```python
from build123d import *

# Parameters (mm, degrees)
SKETCH1_W               = 12
SKETCH1_H               = 12
SKETCH1_R               = 5.5
BOSS_EXTRUDE1_DEPTH     = 2
BOSS_EXTRUDE1_2_DEPTH   = 2
BOSS_EXTRUDE1_3_DEPTH   = 2
BOSS_EXTRUDE1_4_DEPTH   = 2
BOSS_EXTRUDE1_5_DEPTH   = 2
BOSS_EXTRUDE1_6_DEPTH   = 2
BOSS_EXTRUDE2_START     = -10
BOSS_EXTRUDE2_OUTLINE_R = 1.7
BOSS_EXTRUDE2_DEPTH     = 10
CUT_EXTRUDE1_DEPTH      = 1


# Read off the part's stored shape, not the designer's step: Boss-Extrude2
with BuildPart() as part:
    # Sketch1 → Boss-Extrude1 (new body)
    with BuildSketch(Plane(origin=(0, 0, 0), x_dir=(1, 0, 0), z_dir=(0, 1, 0))):
        with Locations((13.686388819, -10.664882883)):
            Rectangle(SKETCH1_W, SKETCH1_H)
        with Locations(Location((13.686388819, -10.664882883, 0), (0, 0, 270))):
            Circle(SKETCH1_R, mode=Mode.SUBTRACT)
    extrude(amount=-BOSS_EXTRUDE1_DEPTH)



with BuildPart() as body_2:
    # Sketch1 → Boss-Extrude1 2 (new body)
    with BuildSketch(Plane(origin=(0, 0, 0), x_dir=(1, 0, 0), z_dir=(0, 1, 0))):
        with Locations((-1.113611181, -10.664882883)):
            Rectangle(SKETCH1_W, SKETCH1_H)
        with Locations(Location((-1.113611181, -10.664882883, 0), (0, 0, 270))):
            Circle(SKETCH1_R, mode=Mode.SUBTRACT)
    extrude(amount=-BOSS_EXTRUDE1_2_DEPTH)


with BuildPart() as body_3:
    # Sketch1 → Boss-Extrude1 3 (new body)
    with BuildSketch(Plane(origin=(0, 0, 0), x_dir=(1, 0, 0), z_dir=(0, 1, 0))):
        with Locations((6.28638882, -23.664882883)):
            Rectangle(SKETCH1_W, SKETCH1_H)
        with Locations(Location((6.28638882, -23.664882883, 0), (0, 0, 270))):
            Circle(SKETCH1_R, mode=Mode.SUBTRACT)
    extrude(amount=-BOSS_EXTRUDE1_3_DEPTH)


with BuildPart() as body_4:
    # Sketch1 → Boss-Extrude1 4 (new body)
    with BuildSketch(Plane(origin=(0, 0, 0), x_dir=(1, 0, 0), z_dir=(0, 1, 0))):
        with Locations((21.08638882, -23.664882883)):
            Rectangle(SKETCH1_W, SKETCH1_H)
        with Locations(Location((21.08638882, -23.664882883, 0), (0, 0, 270))):
            Circle(SKETCH1_R, mode=Mode.SUBTRACT)
    extrude(amount=-BOSS_EXTRUDE1_4_DEPTH)


with BuildPart() as body_5:
    # Sketch1 → Boss-Extrude1 5 (new body)
    with BuildSketch(Plane(origin=(0, 0, 0), x_dir=(1, 0, 0), z_dir=(0, 1, 0))):
        with Locations((35.88638882, -23.664882883)):
            Rectangle(SKETCH1_W, SKETCH1_H)
        with Locations(Location((35.88638882, -23.664882883, 0), (0, 0, 270))):
            Circle(SKETCH1_R, mode=Mode.SUBTRACT)
    extrude(amount=-BOSS_EXTRUDE1_5_DEPTH)


with BuildPart() as body_6:
    # Sketch1 → Boss-Extrude1 6 (new body)
    with BuildSketch(Plane(origin=(0, 0, 0), x_dir=(1, 0, 0), z_dir=(0, 1, 0))):
        with Locations((28.486388819, -10.664882883)):
            Rectangle(SKETCH1_W, SKETCH1_H)
        with Locations(Location((28.486388819, -10.664882883, 0), (0, 0, 270))):
            Circle(SKETCH1_R, mode=Mode.SUBTRACT)
    extrude(amount=-BOSS_EXTRUDE1_6_DEPTH)


with BuildPart() as part_1:
    add(part.part)

    add(body_2.part)  # Boss-Extrude2 merges body 2

    add(body_3.part)  # Boss-Extrude2 merges body 3

    add(body_4.part)  # Boss-Extrude2 merges body 4

    add(body_5.part)  # Boss-Extrude2 merges body 5

    add(body_6.part)  # Boss-Extrude2 merges body 6
    # Boss-Extrude2 outline → Boss-Extrude2 (add)
    with BuildSketch(Plane(origin=(0, 0, 0), x_dir=(1, 0, 0), z_dir=(0, 1, 0)).offset(BOSS_EXTRUDE2_START)):
        Polygon((22.486388819, -4.664882883), (25.986388819, -4.664882883), (25.986388819, -4.164882883), (16.186388819, -4.164882883), (16.186388819, -4.664882883), (19.686388819, -4.664882883), (19.686388819, -16.664882883), (7.686388819, -16.664882883), (7.686388819, -4.664882883), (11.186388819, -4.664882883), (11.186388819, -4.164882883), (1.386388819, -4.164882883), (1.386388819, -4.664882883), (4.886388819, -4.664882883), (4.886388819, -16.664882883), (-7.113611181, -16.664882883), (-7.113611181, -4.664882883), (-3.613611181, -4.664882883), (-3.613611181, -4.164882883), (-18.613611181, -4.164883527), (-18.613611181, -30.164882449), (3.78638882, -30.164882883), (3.78638882, -29.664882883), (0.28638882, -29.664882883), (0.28638882, -17.664882883), (12.28638882, -17.664882883), (12.28638882, -29.664882883), (8.78638882, -29.664882883), (8.78638882, -30.164882883), (18.58638882, -30.164882883), (18.58638882, -29.664882883), (15.08638882, -29.664882883), (15.08638882, -17.664882883), (27.08638882, -17.664882883), (27.08638882, -29.664882883), (23.58638882, -29.664882883), (23.58638882, -30.164882883), (33.38638882, -30.164882883), (33.38638882, -29.664882883), (29.88638882, -29.664882883), (29.88638882, -17.664882883), (41.88638882, -17.664882883), (41.88638882, -29.664882883), (38.38638882, -29.664882883), (38.38638882, -30.164882883), (53.38638882, -30.164882883), (53.38638882, -4.164882883), (30.986388819, -4.164882883), (30.986388819, -4.664882883), (34.486388819, -4.664882883), (34.486388819, -16.664882883), (22.486388819, -16.664882883), align=None)
        with Locations((-13.613611181, -17.164882988)):
            Circle(BOSS_EXTRUDE2_OUTLINE_R, mode=Mode.SUBTRACT)
        with Locations((48.386388819, -17.164882988)):
            Circle(BOSS_EXTRUDE2_OUTLINE_R, mode=Mode.SUBTRACT)
    extrude(amount=BOSS_EXTRUDE2_DEPTH)

    # Sketch2 → Cut-Extrude1 (cut)
    with BuildSketch(Plane.XZ.offset(10)):
        Polygon((-11.090813446, 25.393846705), (-9.544018575, 25.393846705), (-9.544018575, 25.068205679), (-10.805877549, 25.068205679), (-10.805877549, 24.091282602), (-9.544018575, 24.091282602), (-9.544018575, 23.765641577), (-10.805877549, 23.765641577), (-10.805877549, 22.218846705), (-11.090813446, 22.218846705), align=None)
        with BuildLine():
            Line((-8.852031395, 24.416923628), (-9.136967293, 24.416923628))
            add(Edge.make_bspline(
                [(-9.136967293, 24.416923628), (-9.135110232, 24.454725076), (-9.131463015, 24.528966114), (-9.114383067, 24.637209944), (-9.089943843, 24.74067394), (-9.055389453, 24.838527362), (-9.012475901, 24.931635423), (-8.961013662, 25.019628294), (-8.90005924, 25.102170301), (-8.830928846, 25.178496252), (-8.755845866, 25.248516405), (-8.674832621, 25.308982233), (-8.589701775, 25.360070406), (-8.500711605, 25.402779818), (-8.406858094, 25.434838107), (-8.30899293, 25.45862488), (-8.206686142, 25.472936279), (-8.136981265, 25.474474599), (-8.101530594, 25.475256961)],
                knots=[0, 0, 0, 0, 1.10065271, 2.161652631, 3.183658789, 4.190468796, 5.17591951, 6.163126047, 7.15150782, 8.156236427, 9.156009102, 10.134482811, 11.092018607, 12.041330605, 13.001268258, 13.972401359, 14.968799086, 16, 16, 16, 16], degree=3))
            add(Edge.make_bspline(
                [(-8.101530594, 25.475256961), (-8.066716198, 25.474441933), (-7.998307154, 25.472840431), (-7.898465184, 25.459087212), (-7.803417209, 25.437546568), (-7.713349021, 25.407324726), (-7.628979234, 25.366698853), (-7.549674044, 25.3178968), (-7.474489308, 25.261454524), (-7.406810297, 25.195002851), (-7.344663683, 25.124062116), (-7.291049494, 25.048326661), (-7.245136124, 24.97010438), (-7.206865872, 24.888798797), (-7.178693517, 24.803644364), (-7.157304714, 24.71588083), (-7.145214846, 24.624599752), (-7.143359355, 24.562817376), (-7.142416011, 24.531406801)],
                knots=[0, 0, 0, 0, 1.111607364, 2.184268762, 3.212621178, 4.221274766, 5.211760367, 6.196651075, 7.1921475, 8.207485113, 9.220403448, 10.201281604, 11.166441695, 12.114753415, 13.065576456, 14.026450734, 14.996634279, 16, 16, 16, 16], degree=3))
            add(Edge.make_bspline(
                [(-7.142416011, 24.531406801), (-7.143946038, 24.48718376), (-7.146979244, 24.399513729), (-7.173155489, 24.270514062), (-7.21359782, 24.145414473), (-7.262649782, 24.044740618), (-7.31219844, 23.964025865), (-7.355904397, 23.896973819), (-7.408203317, 23.825466998), (-7.468616685, 23.748785207), (-7.536233124, 23.666693885), (-7.611539287, 23.579159348), (-7.695110449, 23.487111285), (-7.753764656, 23.424241012), (-7.784157797, 23.391663211)],
                knots=[0, 0, 0, 0, 1.184203166, 2.347625244, 3.513805382, 4.700623107, 5.337941753, 6.051866363, 6.845199593, 7.711357327, 8.668078039, 9.695487809, 10.805859518, 12, 12, 12, 12], degree=3))
            Line((-7.784157797, 23.391663211), (-8.578543815, 22.544487731))
            Line((-8.578543815, 22.544487731), (-7.101710882, 22.544487731))
            Line((-7.101710882, 22.544487731), (-7.101710882, 22.218846705))
            Line((-7.101710882, 22.218846705), (-9.259082677, 22.218846705))
            Line((-9.259082677, 22.218846705), (-8.027752549, 23.532859125))
            add(Edge.make_bspline(
                [(-8.027752549, 23.532859125), (-7.997773395, 23.564154017), (-7.940189574, 23.624265101), (-7.858743951, 23.712024786), (-7.785592869, 23.793440441), (-7.720262805, 23.868358238), (-7.664170983, 23.937874018), (-7.614394029, 23.999736356), (-7.574510957, 24.056663607), (-7.531226277, 24.122649736), (-7.489303594, 24.203215195), (-7.453278814, 24.301670756), (-7.431312487, 24.403023335), (-7.428677386, 24.471514469), (-7.427351908, 24.505966096)],
                knots=[0, 0, 0, 0, 1.329631726, 2.553950428, 3.673215718, 4.687767853, 5.603093632, 6.413772471, 7.123043292, 7.734684054, 8.834405432, 9.900288307, 10.943827018, 12, 12, 12, 12], degree=3))
            add(Edge.make_bspline(
                [(-7.427351908, 24.505966096), (-7.427928617, 24.527629936), (-7.4290652, 24.570325205), (-7.439096111, 24.632923286), (-7.454254927, 24.693307081), (-7.475976697, 24.751662329), (-7.504648526, 24.807402313), (-7.539549378, 24.860594884), (-7.579817506, 24.912019874), (-7.626400444, 24.960237509), (-7.677573751, 25.004398317), (-7.731634249, 25.043518023), (-7.7888297, 25.076210645), (-7.848918954, 25.103010817), (-7.911734487, 25.124034199), (-7.977397792, 25.138601624), (-8.045727435, 25.147747878), (-8.092384963, 25.148985376), (-8.116158999, 25.149615936)],
                knots=[0, 0, 0, 0, 0.991446411, 1.95395049, 2.89581595, 3.838931463, 4.798493298, 5.75982156, 6.748411868, 7.785213223, 8.824556874, 9.840280684, 10.836137867, 11.835679398, 12.848801643, 13.863922112, 14.911575587, 16, 16, 16, 16], degree=3))
            add(Edge.make_bspline(
                [(-8.116158999, 25.149615936), (-8.140988255, 25.148967299), (-8.189748813, 25.147693485), (-8.26133965, 25.138782925), (-8.329634605, 25.123410627), (-8.394805474, 25.102386072), (-8.456962527, 25.07566296), (-8.515803481, 25.042378306), (-8.571196245, 25.002660423), (-8.623244948, 24.957629347), (-8.671200129, 24.907493737), (-8.713334081, 24.851604699), (-8.75014958, 24.790982687), (-8.782270813, 24.725791273), (-8.808356332, 24.655438916), (-8.828289118, 24.580175355), (-8.844061472, 24.500327387), (-8.84933063, 24.445186632), (-8.852031395, 24.416923628)],
                knots=[0, 0, 0, 0, 1.031018746, 2.02475058, 2.990194455, 3.934040569, 4.864654155, 5.795059489, 6.735614925, 7.690564532, 8.649604399, 9.611025574, 10.590972636, 11.591080095, 12.624614302, 13.701020113, 14.821632451, 16, 16, 16, 16], degree=3))
        make_face()
    extrude(amount=-CUT_EXTRUDE1_DEPTH, mode=Mode.SUBTRACT)


solid = part_1.part
```
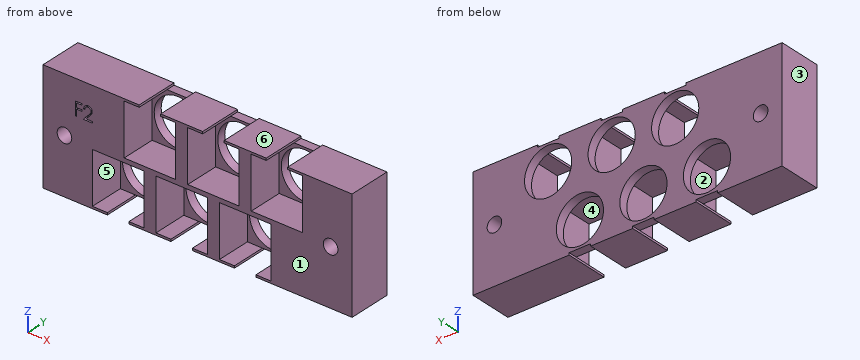
For this review, take the finished solid that the model builds, in its own axes (mm). Face numbers are marked on the shaded views. A direction names the side the tool comes from. Round coordinates to 2 decimals unless told otherwise and drop trailing zeros. Loops run counter-clockwise (first coordinate to the right, second up) from the corner with the lowest first, then second, coordinate; pieces in that order, holes last.
(1) Wall thickness on line 1 along X through (y, z) = (-5, 22); line 2 along Z through (x, y) = (3, -6.25); line 3 along X through (y, z) = (-3.25, 12.5): over which ranges is each line inside the solid? List them lowest first.
Returned:
line 1: x = -18.61 to 0.29, 12.29 to 15.09, 27.09 to 29.89, 41.89 to 53.39
line 2: z = 4.16 to 4.66, 16.66 to 17.66, 29.66 to 30.16
line 3: x = -18.61 to -7.11, 4.89 to 7.69, 19.69 to 22.49, 34.49 to 53.39
(2) Clearance check with flat-ended pins moving along their axes: P1, Ø3, axis at x = -1, z = 15, coming from the -Y side; P2, Ø1, axis at x = 36.5, y = -0.5, coming from the +Z side. State where each tip first meets the part, or that it passes through.
Returned:
P1: stops at y = -2
P2: stops at z = 29.66
(3) Tool access review of the marked faces 1 and 2: name each direction out of +Z, -Z, +X, -X, +Y, -Y from which nothing blocks a thin tool from reaching the whole face with its end or side.
Returned:
face 1: +Z, -Z, +X, -X, -Y
face 2: -Y
(4) We need section A-A (z = 28). Give the boundary of the cut face in (x, y).
Returned:
outline: (-18.61, -10) - (0.29, -10) - (0.29, -2) - (2.9, -2) - (2.9, 0) - (-18.61, 0) - close; (9.67, -2) - (12.29, -2) - (12.29, -10) - (15.09, -10) - (15.09, -2) - (17.7, -2) - (17.7, 0) - (9.67, 0) - close; (24.47, -2) - (27.09, -2) - (27.09, -10) - (29.89, -10) - (29.89, -2) - (32.5, -2) - (32.5, 0) - (24.47, 0) - close; (39.27, -2) - (41.89, -2) - (41.89, -10) - (53.39, -10) - (53.39, 0) - (39.27, 0) - close
(5) Mouldability with a two-part tool opening along X and no side actions: class the marked faces 3, 4, 5 and 6 as released by +X, released by -X, zero draft, split by the parting line, or undercut.
Returned:
face 3: released by -X
face 4: undercut
face 5: undercut
face 6: zero draft
(6) We need section C-C (x = 17.5). Give the boundary of the cut face in (y, z).
Returned:
outline: (-10, 4.16) - (0, 4.16) - (0, 6.7) - (-2, 6.7) - (-2, 4.66) - (-10, 4.66) - close; (-10, 16.66) - (-2, 16.66) - (-2, 14.63) - (0, 14.63) - (0, 19.5) - (-2, 19.5) - (-2, 17.66) - (-10, 17.66) - close; (-10, 29.66) - (-2, 29.66) - (-2, 27.83) - (0, 27.83) - (0, 30.16) - (-10, 30.16) - close
(7) We need section D-D (z = 7.75). Give the boundary of the cut face in (x, y), plus the area to 3 significant figures.
Returned:
outline: (-18.61, -10) - (-7.11, -10) - (-7.11, -2) - (-5.78, -2) - (-5.78, 0) - (-18.61, 0) - close; (3.55, -2) - (4.89, -2) - (4.89, -10) - (7.69, -10) - (7.69, -2) - (9.02, -2) - (9.02, 0) - (3.55, 0) - close; (18.35, -2) - (19.69, -2) - (19.69, -10) - (22.49, -10) - (22.49, -2) - (23.82, -2) - (23.82, 0) - (18.35, 0) - close; (33.15, -2) - (34.49, -2) - (34.49, -10) - (53.39, -10) - (53.39, 0) - (33.15, 0) - close
area: 376 mm2
(8) We need section B-B (x = 48). Give the boundary of the cut face in (y, z).
Returned:
outline: (-10, 4.16) - (0, 4.16) - (0, 15.51) - (-10, 15.51) - close; (-10, 18.82) - (0, 18.82) - (0, 30.16) - (-10, 30.16) - close
